from build123d import *

# Parameters (mm, degrees)
SKETCH1_W           = 142.75
SKETCH1_H           = 130
BOSS_EXTRUDE1_DEPTH = 4
CHAMFER4_SIZE       = 10
CHAMFER5_SIZE       = 10
SKETCH11_R          = 23.5
SKETCH11_R_2        = 2.75
SKETCH11_R_3        = 13
BOSS_EXTRUDE3_DEPTH = 20
CUT_EXTRUDE3_REACH  = 177.695
FILLET5_R           = 20
FILLET8_R           = 10
FILLET9_R           = 50
BOSS_EXTRUDE5_DEPTH = 2


with BuildPart() as part:
    # Sketch1 → Boss-Extrude1 (new body)
    with BuildSketch(Plane(origin=(0, 0, 0), x_dir=(1, 0, 0), z_dir=(0, 1, 0))):
        with Locations((-0.404975067, 0.207290513)):
            Rectangle(SKETCH1_W, SKETCH1_H)
    extrude(amount=BOSS_EXTRUDE1_DEPTH)

    # Chamfer4
    # the kernel refuses this chamfer: 10 mm, written as the material it takes off along each edge
    with BuildSketch(Plane(origin=(-97.496804946, 4, -65.207290513), x_dir=(0, -1, 0), z_dir=(1, 0, 0)), Plane(origin=(96.686854813, 4, 64.792709487), x_dir=(0, -1, 0), z_dir=(-1, 0, 0))) as chamfer4_piece_1:
        Polygon((CHAMFER4_SIZE, 0), (0, -CHAMFER4_SIZE), (0, 0), align=None)
    extrude(amount=194.183659759, mode=Mode.SUBTRACT)

    # Chamfer5
    # the kernel refuses this chamfer: 10 mm, written as the material it takes off along each edge
    with BuildSketch(Plane(origin=(70.970024933, 4, -80.924120393), x_dir=(-1, 0, 0), z_dir=(0, 0, 1))) as chamfer5_piece_1:
        Polygon((CHAMFER5_SIZE, 0), (0, CHAMFER5_SIZE), (0, 0), align=None)
    extrude(amount=161.433659759, mode=Mode.SUBTRACT)

    # Sketch11 → Boss-Extrude3 (add)
    # profile 1 of 2: a face of its own
    with BuildSketch(Plane(origin=(0, 0, 54.792709487), x_dir=(-1, 0, 0), z_dir=(0, 0, -1))):
        with Locations((117.047641156, 67.733126253)):
            Circle(SKETCH11_R)
        with Locations((99.047641156, 67.733126253)):
            Circle(SKETCH11_R_2, mode=Mode.SUBTRACT)
        with Locations((117.047641156, 85.733126253)):
            Circle(SKETCH11_R_2, mode=Mode.SUBTRACT)
        with Locations((135.047641156, 67.733126253)):
            Circle(SKETCH11_R_2, mode=Mode.SUBTRACT)
        with Locations((117.047641156, 49.733126253)):
            Circle(SKETCH11_R_2, mode=Mode.SUBTRACT)
        with Locations((117.047641156, 67.733126253)):
            Circle(SKETCH11_R_3, mode=Mode.SUBTRACT)
    # profile 2 of 2: a face of its own
    with BuildSketch(Plane(origin=(0, 0, 54.792709487), x_dir=(-1, 0, 0), z_dir=(0, 0, -1))):
        Polygon((65.279975067, 4), (71.779975067, 4), (110.625146065, 55.02727289), (106.509975067, 58.16), align=None)
    boss_extrude3 = extrude(amount=BOSS_EXTRUDE3_DEPTH)

    # Sketch12 → Cut-Extrude3 (cut, up to next)
    with BuildSketch(Plane(origin=(0, 4, 0), x_dir=(1, 0, 0), z_dir=(0, 1, 0)), mode=Mode.PRIVATE) as cut_extrude3_sk1:
        with BuildLine():
            Line((-62.033374936, -22.292709487), (12.966625064, -22.292709487))
            ThreePointArc((12.966625064, -22.292709487), (20.037692876, -19.363777299), (22.966625064, -12.292709487))
            Line((22.966625064, -12.292709487), (22.966625064, 22.707290513))
            Line((22.966625064, 22.707290513), (-62.033374936, 22.707290513))
            ThreePointArc((-62.033374936, 22.707290513), (-67.848507835, 20.84265955), (-71.495025362, 15.944136388))
            ThreePointArc((-71.495025362, 15.944136388), (-71.630244869, 15.572907696), (-71.779975067, 15.207290513))
            Line((-71.779975067, 15.207290513), (-71.779975067, -14.792709487))
            ThreePointArc((-71.779975067, -14.792709487), (-71.630247327, -15.158320315), (-71.495029773, -15.529542467))
            ThreePointArc((-71.495029773, -15.529542467), (-67.848513378, -20.428074562), (-62.033374936, -22.292709487))
        make_face()
    cut_extrude3_tool1 = extrude(cut_extrude3_sk1.sketch, amount=-CUT_EXTRUDE3_REACH, mode=Mode.PRIVATE) & part.part
    add(cut_extrude3_tool1.solids().sort_by_distance((-24.222891, 4, -0.310755))[0], mode=Mode.SUBTRACT)

    # Fillet5
    # the kernel refuses this fillet: 20 mm, written as the material it takes off along each edge
    with BuildSketch(Plane(origin=(-71.779975067, 0, 14.792709487), x_dir=(1, 0, 0), z_dir=(0, 0, -1))) as fillet5_piece_1:
        with BuildLine():
            CenterArc((12, -20), FILLET5_R, 90, 36.869897646)
            Line((0, -4), (-0.24, -3.68))
            ThreePointArc((-0.24, -3.68), (-0.4, -2), (-0.4, 0))
            Line((-0.4, 0), (0, 0.4))
            Line((0, 0.4), (12, 0.4))
            Line((12, 0.4), (12, 0))
        make_face()
    extrude(amount=104, mode=Mode.SUBTRACT)
    with BuildSketch(Plane(origin=(-71.779975067, 0, 88.792709487), x_dir=(0, 1, 0), z_dir=(0, 0, -1))) as fillet5_piece_2:
        with BuildLine():
            CenterArc((20, 12), FILLET5_R, 180, 36.869897646)
            Line((0, 12), (-0.4, 12))
            Line((-0.4, 12), (-0.4, 0))
            Line((-0.4, 0), (0, -0.4))
            ThreePointArc((0, -0.4), (2, -0.4), (3.68, -0.24))
            Line((3.68, -0.24), (4, 0))
        make_face()
    extrude(amount=104, mode=Mode.SUBTRACT)

    # Mirror3: Boss-Extrude3 across plane
    add(boss_extrude3.mirror(Plane.XY.offset(-0.207290513)))

    # Fillet8
    # the kernel refuses this fillet: 10 mm, written as the material it adds along each edge
    with BuildSketch(Plane(origin=(-40.279975067, 4, -35.207290513), x_dir=(0, 0, 1), z_dir=(-1, 0, 0))) as fillet8_piece_1_section:
        with BuildLine():
            CenterArc((FILLET8_R, FILLET8_R), FILLET8_R, 180, 90)
            Line((0, FILLET8_R), (0, 0))
            Line((0, 0), (FILLET8_R, 0))
        make_face()
    fillet8_piece_1 = extrude(amount=56.5, mode=Mode.PRIVATE)
    fillet8_piece_1 = split(fillet8_piece_1, bisect_by=Plane(origin=(-56.107555829, -8.048950422, -35.207290513), z_dir=(-0.7956778434191335, -0.6057200421744992, 0)), keep=Keep.TOP, mode=Mode.PRIVATE)
    fillet8_piece_1 = split(fillet8_piece_1, bisect_by=Plane(origin=(-60.222726828, -11.181677532, -35.207290513), z_dir=(0.7956778434191335, 0.605720042174499, 0)), keep=Keep.TOP, mode=Mode.PRIVATE)
    add(fillet8_piece_1)
    with BuildSketch(Plane(origin=(-65.279975067, 4, -55.207290513), x_dir=(1, 0, 0), z_dir=(0, 0, 1))) as fillet8_piece_2:
        with BuildLine():
            CenterArc((FILLET8_R * 0.495527129587, FILLET8_R), FILLET8_R, 217.280673383, 52.719326617)
            Line((-FILLET8_R * 0.300150713832, FILLET8_R * 0.394279957825), (0, 0))
            Line((0, 0), (FILLET8_R * 0.495527129587, 0))
        make_face()
    extrude(amount=20)
    with BuildSketch(Plane(origin=(-65.279975067, 4, 54.792709487), x_dir=(1, 0, 0), z_dir=(0, 0, -1))) as fillet8_piece_3:
        with BuildLine():
            CenterArc((FILLET8_R * 0.495527129587, -FILLET8_R), FILLET8_R, 90, 52.719326617)
            Line((-FILLET8_R * 0.300150713832, -FILLET8_R * 0.394279957825), (0, 0))
            Line((0, 0), (FILLET8_R * 0.495527129587, 0))
        make_face()
    extrude(amount=20)
    with BuildSketch(Plane(origin=(-40.279975067, 4, 34.792709487), x_dir=(0, 0, -1), z_dir=(-1, 0, 0))) as fillet8_piece_4_section:
        with BuildLine():
            CenterArc((FILLET8_R, -FILLET8_R), FILLET8_R, 90, 90)
            Line((0, -FILLET8_R), (0, 0))
            Line((0, 0), (FILLET8_R, 0))
        make_face()
    fillet8_piece_4 = extrude(amount=56.5, mode=Mode.PRIVATE)
    fillet8_piece_4 = split(fillet8_piece_4, bisect_by=Plane(origin=(-56.107555829, -8.048950422, 34.792709487), z_dir=(-0.7956778434191335, -0.6057200421744992, 0)), keep=Keep.TOP, mode=Mode.PRIVATE)
    fillet8_piece_4 = split(fillet8_piece_4, bisect_by=Plane(origin=(-60.222726828, -11.181677532, 34.792709487), z_dir=(0.7956778434191335, 0.605720042174499, 0)), keep=Keep.TOP, mode=Mode.PRIVATE)
    add(fillet8_piece_4)
    with BuildSketch(Plane(origin=(-65.279975067, 4, -55.207290513), x_dir=(1, 0, 0), z_dir=(0, 0, 1))) as fillet8_piece_5a_section:
        with BuildLine():
            CenterArc((FILLET8_R * 0.495527129587, FILLET8_R), FILLET8_R, 217.280673383, 52.719326617)
            Line((-FILLET8_R * 0.300150713832, FILLET8_R * 0.394279957825), (0, 0))
            Line((0, 0), (FILLET8_R * 0.495527129587, 0))
        make_face()
    fillet8_piece_5a = extrude(amount=32.38817824, mode=Mode.PRIVATE)
    fillet8_piece_5a = split(fillet8_piece_5a, bisect_by=Plane(origin=(-65.279975067, 4, -35.207290513), z_dir=(0, 0, 1)), keep=Keep.TOP, mode=Mode.PRIVATE)
    with BuildSketch(Plane(origin=(-40.279975067, 4, -35.207290513), x_dir=(0, 0, 1), z_dir=(-1, 0, 0))) as fillet8_piece_5b_section:
        with BuildLine():
            CenterArc((FILLET8_R, FILLET8_R), FILLET8_R, 180, 90)
            Line((0, FILLET8_R), (0, 0))
            Line((0, 0), (FILLET8_R, 0))
        make_face()
    fillet8_piece_5b = extrude(amount=56.5, mode=Mode.PRIVATE)
    fillet8_piece_5b = split(fillet8_piece_5b, bisect_by=Plane(origin=(-56.107555829, -8.048950422, -35.207290513), z_dir=(0.7956778434191335, 0.6057200421744992, 0)), keep=Keep.TOP, mode=Mode.PRIVATE)
    fillet8_piece_5b = fillet8_piece_5b & Plane(origin=(-59.779975067, 20, -35.207290513), x_dir=(1, 0, 0), z_dir=(0, 0, 1)) * Cylinder(20, 154, mode=Mode.PRIVATE)
    fillet8_piece_5 = fillet8_piece_5a & fillet8_piece_5b
    add(fillet8_piece_5)
    with BuildSketch(Plane(origin=(-40.279975067, 4, 34.792709487), x_dir=(0, 0, -1), z_dir=(-1, 0, 0))) as fillet8_piece_6a_section:
        with BuildLine():
            CenterArc((FILLET8_R, -FILLET8_R), FILLET8_R, 90, 90)
            Line((0, -FILLET8_R), (0, 0))
            Line((0, 0), (FILLET8_R, 0))
        make_face()
    fillet8_piece_6a = extrude(amount=56.5, mode=Mode.PRIVATE)
    fillet8_piece_6a = fillet8_piece_6a & Plane(origin=(-59.779975067, 20, 34.792709487), x_dir=(0, 1, 0), z_dir=(0, 0, 1)) * Cylinder(20, 154, mode=Mode.PRIVATE)
    fillet8_piece_6a = split(fillet8_piece_6a, bisect_by=Plane(origin=(-56.107555829, -8.048950422, 34.792709487), z_dir=(0.7956778434191335, 0.6057200421744992, 0)), keep=Keep.TOP, mode=Mode.PRIVATE)
    with BuildSketch(Plane(origin=(-65.279975067, 4, 54.792709487), x_dir=(1, 0, 0), z_dir=(0, 0, -1))) as fillet8_piece_6b_section:
        with BuildLine():
            CenterArc((FILLET8_R * 0.495527129587, -FILLET8_R), FILLET8_R, 90, 52.719326617)
            Line((-FILLET8_R * 0.300150713832, -FILLET8_R * 0.394279957825), (0, 0))
            Line((0, 0), (FILLET8_R * 0.495527129587, 0))
        make_face()
    fillet8_piece_6b = extrude(amount=32.38817824, mode=Mode.PRIVATE)
    fillet8_piece_6b = split(fillet8_piece_6b, bisect_by=Plane(origin=(-65.279975067, 4, 34.792709487), z_dir=(0, 0, -1)), keep=Keep.TOP, mode=Mode.PRIVATE)
    fillet8_piece_6 = fillet8_piece_6a & fillet8_piece_6b
    add(fillet8_piece_6)

    # Fillet9
    fillet9_edges = [part.edges().sort_by_distance(p)[0] for p in [
        (-104.957249904, 47.581887101, -45.207290513),
        (-100.842078905, 50.714614211, -45.207290513),
        (-104.957249904, 47.581887101, 44.792709487),
        (-100.842078905, 50.714614211, 44.792709487),
    ]]
    fillet(fillet9_edges, radius=FILLET9_R)

    # Sketch14 → Boss-Extrude5 (add)
    with BuildSketch(Plane(origin=(0, 4, 0), x_dir=(1, 0, 0), z_dir=(0, 1, 0))):
        with BuildLine():
            Line((-71.779975067, 15.207290513), (-22.033374936, 15.207290513))
            ThreePointArc((-22.033374936, 15.207290513), (-7.033374936, 0.207290513), (-22.033374936, -14.792709487))
            Line((-22.033374936, -14.792709487), (-71.779975067, -14.792709487))
            ThreePointArc((-71.779975067, -14.792709487), (-71.630247327, -15.158320315), (-71.495029773, -15.529542467))
            ThreePointArc((-71.495029773, -15.529542467), (-67.848513378, -20.428074562), (-62.033374936, -22.292709487))
            Line((-62.033374936, -22.292709487), (12.966625064, -22.292709487))
            ThreePointArc((12.966625064, -22.292709487), (20.037692876, -19.363777299), (22.966625064, -12.292709487))
            Line((22.966625064, -12.292709487), (22.966625064, 22.707290513))
            Line((22.966625064, 22.707290513), (-62.033374936, 22.707290513))
            ThreePointArc((-62.033374936, 22.707290513), (-67.848507835, 20.84265955), (-71.495025362, 15.944136388))
            ThreePointArc((-71.495025362, 15.944136388), (-71.630244869, 15.572907696), (-71.779975067, 15.207290513))
        make_face()
    extrude(amount=-BOSS_EXTRUDE5_DEPTH)


solid = part.part
Model file for the job. Use its own axes, mm. A direction names the side the tool comes from. Round coordinates to 2 decimals unless told otherwise and drop trailing zeros. Loops run counter-clockwise (first coordinate to the right, second up) from the corner with the lowest first, then second, coordinate; pieces in that order, holes last.
1. Band-saw the part on C-C, the plane z = 45.5. List the corners of the cut face in (x, y), and give its area (3 significant figures).
Check values:
outline: (-120.48, 44.49) arc R50 cw to (-88, 25.31) - (-71.78, 4) arc R20 ccw to (-59.78, 0) - (64.97, 0) - (60.97, 4) - (-60.32, 4) arc R10 cw to (-68.28, 7.94) - (-83.89, 28.44) arc R50 cw to (-93.72, 64.85) arc R23.5 ccw (long way) to start; hole circle Ø5.5 at (-135.05, 67.73); hole circle Ø26 at (-117.05, 67.73); hole circle Ø5.5 at (-117.05, 49.73); hole circle Ø5.5 at (-117.05, 85.73); hole circle Ø5.5 at (-99.05, 67.73)
area: 2,110 mm2
2. Wall check: probe 1 along Z at (x, y) = (-97, 78.5); probe 2 along Y at (x, z) = (40, 39); probe 3 along Y at (x, z) = (-98, 40.5). Give the ranges that are in metal, low to high.
Check values:
probe 1: z = -55.21 to -35.21, 34.79 to 54.79
probe 2: y = 0 to 4
probe 3: y = 35.18 to 65.19, 70.28 to 81.5
3. Band-saw the part on B-B, the plane y = 35.5. List the corners of the cut face in (x, z), and give its area (3 significant figures).
Check values:
outline: (-98.43, -55.21) - (-88.38, -55.21) - (-88.38, -35.21) - (-98.43, -35.21) - close; (-98.43, 34.79) - (-88.38, 34.79) - (-88.38, 54.79) - (-98.43, 54.79) - close
area: 402 mm2
4. Drop flat-ended pins along their axis: P1, Ø0.6, axis at y = 0.5, z = -13, coming from the -X side; P2, Ø5, axis at y = 57.5, z = -35.5, coming from the +X side; P3, Ø1, axis at x = -65, z = -33, coming from the -Y side. Give the stop position or say it passes through.
Check values:
P1: stops at x = 22.97
P2: stops at x = -93.96
P3: stops at y = 0.56
5. Tool access for faces 5 (the cylindrical face through (-101.67, 68.56, -45.35)), 6 (the cylindrical face through (-66.02, 1, -41.79)): list every direction of +Z, -Z, +X, -X, +Y, -Y with a clear straight run to the whole face (end or side of a thin tool).
Check values:
face 5: +Z, -Z
face 6: -Z, -X, -Y
6. Band-saw the part on A-A, the plane x = -16. List the corners of the cut face in (y, z).
Check values:
outline: (0, -59.21) - (4, -55.21) - (4, -13.94) - (2, -13.94) - (2, -22.71) - (0, -22.71) - close; (0, 22.29) - (2, 22.29) - (2, 13.53) - (4, 13.53) - (4, 54.79) - (0, 58.79) - close
7. Mould opens along Y. For faces 1 (the cylindrical face through (-101.67, 68.56, 44.93)), 2 (the cylindrical face through (20, 1, 19.4)), 3 (the cylindrical face through (-64.707, 5.011, 43.336)), 4 (the flat face through (-4, 2, -1)) say: +Y half, -Y half, draft (parallel to the pull), parting line (faces both ways), or undercut.
Check values:
face 1: undercut
face 2: draft
face 3: +Y half
face 4: -Y half
8. Band-saw the part on D-D, the plane y = 77.5. List the corners of the cut face in (x, z), and give its area (3 significant figures).
Check values:
outline: (-138.42, -55.21) - (-125.63, -55.21) - (-125.63, -35.21) - (-138.42, -35.21) - close; (-138.42, 34.79) - (-125.63, 34.79) - (-125.63, 54.79) - (-138.42, 54.79) - close; (-108.47, -55.21) - (-95.67, -55.21) - (-95.67, -35.21) - (-108.47, -35.21) - close; (-108.47, 34.79) - (-95.67, 34.79) - (-95.67, 54.79) - (-108.47, 54.79) - close
area: 1,020 mm2
